Read the model definition and answer for the solid it produces. Units are mm, in the model's axes. A direction names the side the tool comes from. Coordinates: 2 decimals unless noted, no trailing zeros. Loops run counter-clockwise (first coordinate to the right, second up) from the corner with the lowest first, then second, coordinate; pieces in that order, holes last. Notation, with made-up numbers: (86.25, 48.5) -> (122.25, 48.5) arc R7 ccw to (122.25, 54.5) -> close; hole circle Ø2 at (61, -27). An arc over 180 degrees is marked (long way). One line per question, with ' | ' between items. Start each with the question number.
Autodesk Inventor part; units mm, degrees
ref_plane "YZ Plane" through (0, 0, 0) normal (1, 0, 0) x (0, 1, 0)
ref_plane "XZ Plane" through (0, 0, 0) normal (0, 1, 0) x (-1, 0, 0)
ref_plane "XY Plane" through (0, 0, 0) normal (0, 0, 1) x (1, 0, 0)
sketch "Sketch1" plane through (0, 0, 0) normal (0, 1, 0) x (-1, 0, 0)
  line L0 (470, 0) -> (470, -30)
  arc A0 (432.7406, -89.4136) -> (470, -30) centre (404, -30) ccw
  arc A1 (20, -184) -> (432.7406, -89.4136) centre (20, 763.8182) ccw
  line L1 (0, 0) -> (0, -191.6842)
  arc A2 (20, -178) -> (430.1278, -84.0124) centre (20, 763.8182) ccw
  arc A3 (430.1278, -84.0124) -> (464, -30) centre (404, -30) ccw
  line L2 (464, -30) -> (464, 0)
  line L3 (464, 0) -> (470, 0)
  line L4 (0, -178) -> (0, -184)
  line L5 (0, -184) -> (20, -184)
  line L6 (0, -178) -> (20, -178)
  point P0 (0, 0)
  point P1 (0, -163.7009)
  point P2 (0, -169.7009)
  dimension "d1" = 30
  dimension "d3" = 947.8182
  dimension "d12" = 184
  dimension "d13" = 6
  dimension "d14" = 40
  dimension "d15" = 60
  dimension "d16" = 940
revolve "Revolution1" add sketch "Sketch1" angle 360 about axis through (0, 0, 0) along (0, 0, -1)
sketch "Sketch2" plane through (0, 0, 0) normal (0, 0, 1) x (1, 0, 0)
  circle A0 centre (0, 0) radius 16.75
  dimension "d8" = 33.5
extrude "Extrusion1" cut sketch "Sketch2" against normal through all
equation "\"d16\" = AA_MAIN_filter_diam"
properties part number "PRS 1604 dished head_D1200 940"
(1) Determine the mould class of faces 1 (the cylindrical face through (61.2, 466, -15.2)), 2 (the flat face through (-346, -311, 0)), 3 (the cylindrical face through (-3.63, -16.35, -180.96)) for opening direction Y: +Y half, -Y half, draft (parallel to the pull), parting line (faces both ways), or undercut.
(2) Find the intervals of material crossed by probe 1 along Y at (x, z) = (0, -10); probe 2 along Y at (x, z) = (-189.5, -60); probe 3 along X at (y, z) = (-292, -20), in increasing order. Write a range as from..to.
(3) Each of these flat-tipped pins is pushed along its axis until it touches: pin 1 Ø12 at (x, y) = (-271, 273.5) entering from -Z; pin 2 Ø2 at (x, y) = (-375.5, 33) entering from +Z; pin 3 Ø5 at (x, z) = (186, -39.5) entering from -Y. Where does it stop, or does it pass through?
(4) Section A-A on z = -63 is taken. Write down the section's boundary in (x, y), plus the area to 3 significant figures.
(5) A tool of negligible diameter and unlimited length cuts with its end or side. For faces 4 (the flat face through (12, -12, -178)), 5 (the flat face through (12, -12, -184)), from which of +Z, -Z, +X, -X, +Y, -Y can it reach the whole face along a straight path? Write none if from no direction.
Working result:
1) face 1: parting line | face 2: draft | face 3: undercut
2) probe 1: y = -470..-464, 464..470 | probe 2: y = -422.21..-414.72, 414.72..422.21 | probe 3: x = -368.29..-360.6, 360.6..368.29
3) pin 1: stops at z = -113.37 | pin 2: stops at z = -107.33 | pin 3: stops at y = -432.02
4) outline: circle Ø922.32 at (0, 0); hole circle Ø908.22 at (0, 0) | area: 20,300 mm2
5) face 4: +Z | face 5: -Z, +X, -X, +Y, -Y
